Verification items for the finished model (mm, model axes). Face numbers are marked on the shaded views. A direction names the side the tool comes from. Give positions to 0.01 mm unless a question says otherwise; leave off trailing zeros. Write each loop counter-clockwise with the first axis right and the second up, starting at its lowest first coordinate (ties: lowest second). Pieces come first, ordered by that corner, then holes. Notation, with made-up numbers: (87, 71) -> (124, 71) arc R34 ccw to (124, 110) -> close; hole circle Ø7 at (-13.5, 5.5). An arc over 180 degrees is marked (long way). Use one line per item in the form item = value. Start each with the question number.
(1) Set-up check for the marked faces 4 and 5: record each of +Z, -Z, +X, -X, +Y, -Y from which the full face is reachable in a straight line by a thin tool's end or side.
(2) Section check A-A, the plane y = 0. Record the cut outline in (x, z) (3 decimals).
(3) Scan lines: L1, parallel to Y at x = 1.55, z = 0; L2, parallel to Z at x = -0.6, y = 0. Record each from-to range of solid material in increasing order.
(4) Section check C-C, the plane x = -0.55. Record the cut outline in (y, z), plus the area to 3 significant figures.
(5) Section check D-D, the plane x = 0.25. Record the cut outline in (y, z), plus the area to 3 significant figures.
(6) Release check for a two-part mould opening along Z. For the marked faces 1, 2 and 3 record: pulls with the +Z half, pulls with the -Z half, needs draft (parallel to the pull), parting line crosses it, or undercut.
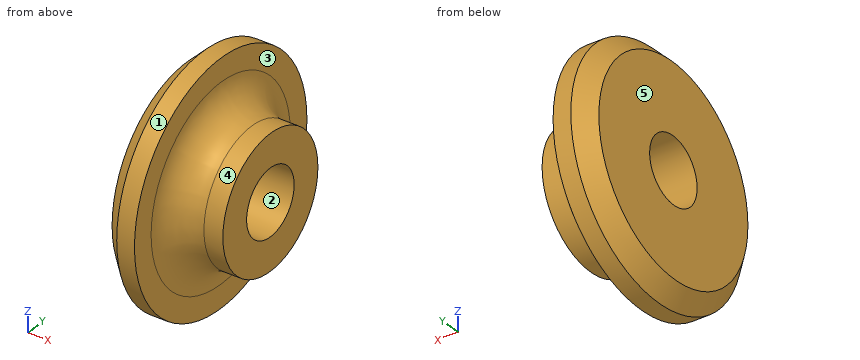
Autodesk Inventor part; units mm, degrees
ref_plane "YZ Plane" through (0, 0, 0) normal (1, 0, 0) x (0, 1, 0)
ref_plane "XZ Plane" through (0, 0, 0) normal (0, 1, 0) x (-1, 0, 0)
ref_plane "XY Plane" through (0, 0, 0) normal (0, 0, 1) x (1, 0, 0)
sketch "스케치1" plane through (0, 0, 0) normal (1, 0, 0) x (0, 1, 0)
  circle A0 centre (0, 0) radius 6.5
  circle A1 centre (0, 0) radius 1.75
  circle A2 centre (0, 0) radius 3.5
  dimension "d0" = 13
  dimension "d1" = 3.5
  dimension "d2" = 7
extrude "돌출1" add sketch "스케치1" against normal blind 2 contours A0 | A2
extrude "돌출2" add sketch "스케치1" along normal blind 2.625 contours A2
fillet "모깎기1" radius 1.625 1 edges at (0, -3.5, 0)
chamfer "모따기1" distance 1 angle 45 1 edges at (-2, -6.5, 0)
move faces "이동1" translate (0.2, 0, 0) faces at (-2, 4.1798, -0.5783)
offset faces "크기2" outward -0.15 faces at (-0.3333, 6.4789, -0.523) (-1.2667, -2.6722, -5.6315)
properties part number "축종아리베어링고정_3D 인쇄"
Completed:
q1.face_4 = +X
q1.face_5 = +Z, -Z, -X, +Y, -Y
q2.outline = (-1.8, -5.488) -> (-0.938, -6.35) -> (0, -6.35) -> (0, -5.125) arc R1.625 cw to (1.625, -3.5) -> (2.625, -3.5) -> (2.625, -1.75) -> (-1.8, -1.75) -> close; (-1.8, 1.75) -> (2.625, 1.75) -> (2.625, 3.5) -> (1.625, 3.5) arc R1.625 cw to (0, 5.125) -> (0, 6.35) -> (-0.938, 6.35) -> (-1.8, 5.488) -> close
q3.L1 = -3.5 to -1.75, 1.75 to 3.5
q3.L2 = -6.35 to -1.75, 1.75 to 6.35
q4.outline = circle Ø12.7 at (0, 0); hole circle Ø3.5 at (0, 0)
q4.area = 117 mm²
q5.outline = circle Ø8.52 at (0, 0); hole circle Ø3.5 at (0, 0)
q5.area = 47.4 mm²
q6.face_1 = parting line crosses it
q6.face_2 = undercut
q6.face_3 = needs draft
